Part model, mm, in its own coordinate system. A direction names the side the tool comes from. Give positions to 0.01 mm unless a question says otherwise; leave off trailing zeros. Order: outer loops, then holes, each group sorted by start corner. A loop starts at its lowest first (then second) coordinate and runs counter-clockwise, first axis right, second up.
1. Mould opens along X. For faces 4 (the flat face through (-1, -48.5, 3)), 5 (the cylindrical face through (-3.088, -29.922, 2.81)), 6 (the flat face through (26.75, -23, 3)), 7 (the flat face through (3.89, -10.11, 4.22)) say: +X half, -X half, draft (parallel to the pull), parting line (faces both ways), or undercut.
2. Which spindle directions (+Z, -Z, +X, -X, +Y, -Y) get a long thin tool onto all of the face, cutting with end or side? Do faces 1 (the cylindrical face through (-13.034, -48.064, 2.81)), 2 (the flat face through (6.644, -10.13, 4.221)), 3 (the cylindrical face through (26.156, -38.438, 2.81)). Say none if no direction does.
3. Slice it at D-D on x = -20.5. List the corners of the cut face in (y, z), and give its area (3 significant figures).
4. Probe line 1 (X direction, y = -32.5, z = 3.95); line 2 (X direction, y = -44, z = 3.7); line 3 (X direction, y = -38, z = 2.9). List the from-to ranges inside material, lowest first.
5. Slice it at C-C on z = 1.9. List the corners of the cut face in (x, y).
6. Slice it at B-B on y = -12.5. List the corners of the cut face in (x, z).
7. Drop a flat-ended pin along its axis: pin 1 Ø9.5 at (x, y) = (-20.5, -44) entering from -Z. Give the stop position or say it passes through.
8. Slice it at A-A on y = -32.5. List the corners of the cut face in (x, z).
from build123d import *

# Parameters (mm, degrees)
SKIZZE2_W                       = 58
SKIZZE2_H                       = 42
AUFSATZ_LINEAR_AUSTRAGEN1_DEPTH = 5.7
SKIZZE1_R                       = 9
SKIZZE1_R_2                     = 8
SKIZZE1_R_3                     = 2.6
SCHNITT_LINEAR_AUSTRAGEN2_DEPTH = 58.976741026
SCHNITT_LINEAR_AUSTRAGEN3_DEPTH = 58.976741026
VERRUNDUNG1_R                   = 1
SCHNITT_LINEAR_AUSTRAGEN4_DEPTH = 3
SKIZZE5_R                       = 1.6
SCHNITT_LINEAR_AUSTRAGEN5_DEPTH = 58.773804618


with BuildPart() as part:
    # Skizze2 → Aufsatz-Linear austragen1 (new body)
    with BuildSketch(Plane.XY):
        with Locations((-2.25, -27.5)):
            Rectangle(SKIZZE2_W, SKIZZE2_H)
    extrude(amount=AUFSATZ_LINEAR_AUSTRAGEN1_DEPTH)

    # Skizze1 → Schnitt-Linear austragen2 (cut, through all)
    with BuildSketch(Plane.XY):
        Circle(SKIZZE1_R)
        with Locations((-20.5, -44)):
            Circle(SKIZZE1_R_2)
        with Locations((19.5, -44)):
            Circle(SKIZZE1_R_2)
        with Locations((11.25, -32.5)):
            Circle(SKIZZE1_R_3)
        with Locations((-2.75, -32.5)):
            Circle(SKIZZE1_R_3)
    extrude(amount=SCHNITT_LINEAR_AUSTRAGEN2_DEPTH, mode=Mode.SUBTRACT)


with BuildPart() as schnitt_linear_austragen2_piece_1:
    # of the separate pieces the step leaves, piece 1, a body of its own (schnitt_linear_austragen2_pieces)
    add(part.part.solids().sort_by_distance((-31.25, -6.5, 0))[0])

    # Verrundung1
    verrundung1_edges = [schnitt_linear_austragen2_piece_1.edges().sort_by_distance(p)[0] for p in [
        (26.75, -6.5, 2.85),
        (-31.25, -48.5, 2.85),
        (-31.25, -6.5, 2.85),
        (-13.885621722, -48.5, 2.85),
        (-27.114378278, -48.5, 2.85),
        (26.75, -40.618062685, 2.85),
        (12.885621722, -48.5, 2.85),
        (-6.224949799, -6.5, 2.85),
        (6.224949799, -6.5, 2.85),
    ]]
    fillet(verrundung1_edges, radius=VERRUNDUNG1_R)

    # Skizze4 → Schnitt-Linear austragen4 (cut)
    with BuildSketch(Plane.XY.offset(5.7)):
        Polygon((2.5, -14.08771324), (5.25, -15.675426481), (8, -14.08771324), (8, -10.91228676), (5.25, -9.324573519), (2.5, -10.91228676), align=None)
    extrude(amount=-SCHNITT_LINEAR_AUSTRAGEN4_DEPTH, mode=Mode.SUBTRACT)

    # Skizze5 → Schnitt-Linear austragen5 (cut, through all)
    with BuildSketch(Plane.XY.offset(2.7)):
        with Locations((5.25, -12.5)):
            Circle(SKIZZE5_R)
    extrude(amount=-SCHNITT_LINEAR_AUSTRAGEN5_DEPTH, mode=Mode.SUBTRACT)


with BuildPart() as schnitt_linear_austragen2_piece_2:
    # of the separate pieces the step leaves, piece 2, a body of its own (schnitt_linear_austragen2_pieces)
    add(part.part.solids().sort_by_distance((26.114378278, -48.5, 0))[0])

    # Skizze3 → Schnitt-Linear austragen3 (cut, through all)
    with BuildSketch(Plane.XY.offset(5.7)):
        with BuildLine():
            Line((26.75, -48.5), (26.75, -47.381937315))
            ThreePointArc((26.75, -47.381937315), (26.454693545, -47.953762474), (26.114378278, -48.5))
            Line((26.114378278, -48.5), (26.75, -48.5))
        make_face()
    extrude(amount=-SCHNITT_LINEAR_AUSTRAGEN3_DEPTH, mode=Mode.SUBTRACT)


solid = schnitt_linear_austragen2_piece_1.part
Data:
1. face 4: draft
1. face 5: undercut
1. face 6: +X half
1. face 7: undercut
2. face 1: +Z, -Z
2. face 2: +Z
2. face 3: +Z, -Z, -Y
3. outline: (-36, 0) - (-6.5, 0) - (-6.5, 5.7) - (-36, 5.7) - close
3. area: 168 mm2
4. line 1: x = -31.25 to -5.35, -0.15 to 8.65, 13.85 to 26.75
4. line 2: x = -31.25 to -28.5, -12.5 to 11.5
4. line 3: x = -31.25 to -25.79, -15.21 to 14.21, 24.79 to 26.63
5. outline: (-31.25, -47.5) arc R1 ccw to (-30.25, -48.5) - (-28.79, -48.5) arc R1 ccw to (-27.87, -47.11) arc R8 cw (long way) to (-13.13, -47.11) arc R1 ccw to (-12.21, -48.5) - (11.21, -48.5) arc R1 ccw to (12.13, -47.11) arc R8 cw to (25.06, -38.24) arc R1 ccw to (26.75, -37.52) - (26.75, -7.5) arc R1 ccw to (25.75, -6.5) - (6.61, -6.5) arc R1 ccw to (5.95, -6.75) arc R9 cw to (-5.95, -6.75) arc R1 ccw to (-6.61, -6.5) - (-30.25, -6.5) arc R1 ccw to (-31.25, -7.5) - close; hole circle Ø5.2 at (-2.75, -32.5); hole circle Ø3.2 at (5.25, -12.5); hole circle Ø5.2 at (11.25, -32.5)
6. outline: (-31.25, 0) - (3.65, 0) - (3.65, 2.7) - (2.5, 2.7) - (2.5, 5.7) - (-31.25, 5.7) - close; (6.85, 0) - (26.75, 0) - (26.75, 5.7) - (8, 5.7) - (8, 2.7) - (6.85, 2.7) - close
7. pin 1: passes through
8. outline: (-31.25, 0) - (-5.35, 0) - (-5.35, 5.7) - (-31.25, 5.7) - close; (-0.15, 0) - (8.65, 0) - (8.65, 5.7) - (-0.15, 5.7) - close; (13.85, 0) - (26.75, 0) - (26.75, 5.7) - (13.85, 5.7) - close
